```python
from build123d import *

# Parameters (mm, degrees)
SKETCH1_W           = 25
SKETCH1_H           = 100
BOSS_EXTRUDE1_DEPTH = 3
SKETCH2_W           = 3
SKETCH2_H           = 100
BOSS_EXTRUDE2_DEPTH = 50
SKETCH3_R           = 1.7
CUT_EXTRUDE1_DEPTH  = 25
SKETCH4_R           = 2.2
CUT_EXTRUDE2_DEPTH  = 25
FILLET1_R           = 5
BOSS_EXTRUDE3_DEPTH = 3
FILLET2_R           = 5


with BuildPart() as part:
    # Sketch1 → Boss-Extrude1 (new body)
    with BuildSketch(Plane(origin=(0, 0, 0), x_dir=(1, 0, 0), z_dir=(0, 1, 0))):
        Rectangle(SKETCH1_W, SKETCH1_H)
    extrude(amount=BOSS_EXTRUDE1_DEPTH)

    # Sketch2 → Boss-Extrude2 (add)
    with BuildSketch(Plane(origin=(0, 3, 0), x_dir=(1, 0, 0), z_dir=(0, 1, 0))):
        with Locations((11, 0)):
            Rectangle(SKETCH2_W, SKETCH2_H)
    extrude(amount=BOSS_EXTRUDE2_DEPTH)

    # Sketch3 → Cut-Extrude1 (cut)
    with BuildSketch(Plane.ZY.offset(-9.5)):
        with Locations((-22.5, 46.5)):
            Circle(SKETCH3_R)
        with Locations((22.5, 46.5)):
            Circle(SKETCH3_R)
    extrude(amount=-CUT_EXTRUDE1_DEPTH, mode=Mode.SUBTRACT)

    # Sketch4 → Cut-Extrude2 (cut)
    with BuildSketch(Plane(origin=(0, 3, 0), x_dir=(1, 0, 0), z_dir=(0, 1, 0))):
        with Locations(Location((-1.5, -1.579280152, 0), (0, 0, 270))):
            Circle(SKETCH4_R)
        with Locations(Location((-1.5, 38.420719848, 0), (0, 0, 270))):
            Circle(SKETCH4_R)
        with Locations(Location((-1.5, -41.579280152, 0), (0, 0, 270))):
            Circle(SKETCH4_R)
    extrude(amount=-CUT_EXTRUDE2_DEPTH, mode=Mode.SUBTRACT)

    # Fillet1
    fillet1_edges = [part.edges().sort_by_distance(p)[0] for p in [
        (9.5, 3, 0),
    ]]
    fillet(fillet1_edges, radius=FILLET1_R)

    # Sketch5 → Boss-Extrude3 (add)
    with BuildSketch(Plane.XY.offset(50)):
        with BuildLine():
            Line((9.5, 53), (-12.5, 3))
            Line((-12.5, 3), (4.5, 3))
            ThreePointArc((4.5, 3), (8.035533906, 4.464466094), (9.5, 8))
            Line((9.5, 8), (9.5, 53))
        make_face()
    boss_extrude3 = extrude(amount=-BOSS_EXTRUDE3_DEPTH)

    # Mirror1: Boss-Extrude3 across plane
    add(boss_extrude3.mirror(Plane.XY))

    # Fillet2
    # the kernel refuses this fillet: 5 mm, written as the material it takes off along each edge
    with BuildSketch(Plane(origin=(25, 53, -50), x_dir=(0, 0, 1), z_dir=(-1, 0, 0))) as fillet2_piece_1:
        with BuildLine():
            CenterArc((FILLET2_R, -FILLET2_R), FILLET2_R, 90, 90)
            Line((0, -FILLET2_R), (0, 0))
            Line((0, 0), (FILLET2_R, 0))
        make_face()
    extrude(amount=28, mode=Mode.SUBTRACT)
    with BuildSketch(Plane(origin=(-3, 53, 50), x_dir=(0, -1, 0), z_dir=(1, 0, 0)), Plane(origin=(-12.5, -12.5, -50), x_dir=(0, 0, 1), z_dir=(0, 1, 0)), Plane(origin=(-12.5, -12.5, 50), x_dir=(1, 0, 0), z_dir=(0, 1, 0))) as fillet2_piece_2:
        with BuildLine():
            CenterArc((FILLET2_R, FILLET2_R), FILLET2_R, 180, 90)
            Line((0, FILLET2_R), (0, 0))
            Line((0, 0), (FILLET2_R, 0))
        make_face()
    extrude(amount=28, mode=Mode.SUBTRACT)


solid = part.part
```
Geometry: final body of the model. Coordinates: model frame, mm. A direction names the side the tool comes from. Give positions to 0.01 mm unless a question says otherwise; leave off trailing zeros. Order: outer loops, then holes, each group sorted by start corner. A loop starts at its lowest first (then second) coordinate and runs counter-clockwise, first axis right, second up. Notation, with made-up numbers: (27.25, 85.5) -> (64.25, 85.5) arc R14 ccw to (64.25, 107.5) -> close; hole circle Ø11 at (-22, 27). An arc over 180 degrees is marked (long way). Write each question's results on one line, items separated by ' | '. Start each with the question number.
1) Draft query along X for faces 3 (the cylindrical face through (11, 45, -21.7)), 4 (the flat face through (12.5, 26, 1)), 5 (the cylindrical face through (-2.343, 1.521, 43.612)). Return one class per face: pulls with the +X half, pulls with the -X half, needs draft (parallel to the pull), parting line crosses it, or undercut.
2) Set-up query: faces 1 (the cylindrical face through (11, 45, 23.3)), 2 (the flat face through (1, 17, 47)). Return all of +Z, -Z, +X, -X, +Y, -Y with unobstructed straight access to the full face (end or side cutting, diameter ignored); none if empty.
3) Section A-A (z = 22.5). Return loops of the section in (x, y), then the cut area to 3 significant figures.
4) Section B-B (x = -1.5). Return loops of the section in (y, z).
5) Line query: line 1 (Z direction, x = 5, y = 20); line 2 (Y direction, x = 11.3, z = -22.5); line 3 (X direction, y = 9.5, z = -18). Output: solid intervals per line, ascending. Write a range as from..to.
6) Section C-C (y = 46.5). Return loops of the section in (x, z).
7) Section D-D (y = 20.5). Return loops of the section in (x, z), then the cut area to 3 significant figures.
8) First-contact query: pin 1 (13.5 mm diameter, centred on x = -4, z = -7.5, fed in from +Y); pin 2 (12 mm diameter, centred on y = 32, z = 16, fed in from -X); pin 3 (8 mm diameter, centred on x = 2, z = -14, fed in from +Y). Flat tips, straight axial feed; report the tip coordinate or a pass-through.
Calculated:
1) face 3: needs draft | face 4: pulls with the +X half | face 5: undercut
2) face 1: +X, -X | face 2: -X, +Y
3) outline: (-12.5, 0) -> (12.5, 0) -> (12.5, 44.8) -> (9.5, 44.8) -> (9.5, 8) arc R5 cw to (4.5, 3) -> (-12.5, 3) -> close; (9.5, 48.2) -> (12.5, 48.2) -> (12.5, 53) -> (9.5, 53) -> close | area: 220 mm2
4) outline: (0, -50) -> (28, -50) -> (28, -47) -> (3, -47) -> (3, -40.62) -> (0, -40.62) -> close; (0, -36.22) -> (3, -36.22) -> (3, -0.62) -> (0, -0.62) -> close; (0, 3.78) -> (3, 3.78) -> (3, 39.38) -> (0, 39.38) -> close; (0, 43.78) -> (3, 43.78) -> (3, 47) -> (28, 47) -> (28, 50) -> (0, 50) -> close
5) line 1: -50..-47, 47..50 | line 2: 0..44.8, 48.2..53 | line 3: 9.5..12.5
6) outline: (6.64, -50) -> (12.5, -50) -> (12.5, -24.2) -> (9.5, -24.2) -> (9.5, -47) -> (6.64, -47) -> close; (6.64, 47) -> (9.5, 47) -> (9.5, 24.2) -> (12.5, 24.2) -> (12.5, 50) -> (6.64, 50) -> close; (9.5, -20.8) -> (12.5, -20.8) -> (12.5, 20.8) -> (9.5, 20.8) -> close
7) outline: (-4.8, -50) -> (12.5, -50) -> (12.5, 50) -> (-4.8, 50) -> (-4.8, 47) -> (9.5, 47) -> (9.5, -47) -> (-4.8, -47) -> close | area: 386 mm2
8) pin 1: y = 3 | pin 2: x = 9.5 | pin 3: y = 3.23
